from build123d import *

# Parameters (mm, degrees)
F1_R     = 4.7625
F2_DEPTH = 3.175
F3_R     = 12.7
F5_DEPTH = 336.55
F6_R     = 3.175


with BuildPart() as f2:
    # F1 (on Front) → F2 (new body)
    with BuildSketch(Plane.XZ):
        with BuildLine():
            Line((0, 438.028063), (0, 0))
            Line((0, 0), (336.55, 0))
            Line((336.55, 0), (336.55, 463.55))
            ThreePointArc((336.55, 463.55), (312.97337, 491.937548), (280.739907, 473.973298))
            Line((280.739907, 473.973298), (255.797312, 409.526661))
            Line((255.797312, 409.526661), (166.350515, 398.862006))
            Line((166.350515, 398.862006), (162.776801, 398.435916))
            Line((162.776801, 398.435916), (159.510839, 399.948027))
            Line((159.510839, 399.948027), (32.464507, 458.769359))
            ThreePointArc((32.464507, 458.769359), (10.552386, 457.288903), (0, 438.028063))
        make_face()
        with Locations((25.4, 419.1)):
            Circle(F1_R, mode=Mode.SUBTRACT)
        with Locations((309.557942, 388.978135)):
            Circle(F1_R, mode=Mode.SUBTRACT)
        with Locations((311.101928, 413.858754)):
            Circle(F1_R, mode=Mode.SUBTRACT)
        with Locations((310.471551, 438.779263)):
            Circle(F1_R, mode=Mode.SUBTRACT)
        with Locations((307.671607, 463.55)):
            Circle(F1_R, mode=Mode.SUBTRACT)
    extrude(amount=F2_DEPTH)

    # F3
    f3_edges = [f2.edges().sort_by_distance(p)[0] for p in [
        (162.776801, -1.5875, 398.435916),
        (255.797312, -1.5875, 409.526661),
    ]]
    fillet(f3_edges, radius=F3_R)

    # F4 (on Right) → F5 (join, through all)
    with BuildSketch(Plane.YZ):
        Polygon((0, 0), (-3.175, 0), (-3.175, -3.175), (50.8, -3.175), (50.8, 0), align=None)
    extrude(amount=F5_DEPTH)

    # F6
    f6_edges = [f2.edges().sort_by_distance(p)[0] for p in [
        (168.275, -3.175, -3.175),
    ]]
    fillet(f6_edges, radius=F6_R)


solid = f2.part
Can you work these out from the model? Positions are in its coordinate system, mm. A direction names the side the tool comes from. Coordinates: 2 decimals unless noted, no trailing zeros. Write each loop counter-clockwise with the first axis right and the second up, starting at its lowest first coordinate (ties: lowest second). Pieces come first, ordered by that corner, then holes. Notation, with made-up numbers: (-3.5, 87.5) -> (23.5, 87.5) arc R16 ccw to (23.5, 109.5) -> close; hole circle Ø7 at (-23.5, 0). An arc over 180 degrees is marked (long way). Write each question's results on one line, items separated by ' | '. Start each with the question number.
Q1. Imagine slicing it at D-D (x = 195). Write out the boundary of the cut face in (y, z) (3 decimals).
Q2. If I drill on probe 1 along Z at (x, y) = (201.5, 41) (3 decimals); probe 2 along X at (y, z) = (-1.7, 463.55), over which ranges is the centre line in solid material (lowest first)?
Q3. Imagine slicing it at B-B (z = 261). Write out the boundary of the cut face in (x, y) (3 decimals), then the cut area to 3 significant figures.
Q4. On a 3-axis mill with a long thin cutter (end or side, diameter ignored), from which of +Z, -Z, +X, -X, +Y, -Y can I reach the whole of each face in a straight line? I mean faces 1 (the face through (303.892, -1.565, 460.652)), 2 (the face through (166, 26, 0)). Say none if no direction works.
Q5. Imagine slicing it at A-A (x = 131.5). Write out the boundary of the cut face in (y, z) (3 decimals), then the cut area to 3 significant figures.
Q6. We'd pull the mould along Z, two halves only. Please class faces 3 (the face through (269.8, -1.57, 445.71)), 4 (the face through (24.37, -1.57, 414.45)), 5 (the face through (166, 0, 195)): +Z half, -Z half, draft (parallel to the pull), parting line (faces both ways), or undercut.
Q7. I'm going to push flat-ended pins straight in: pin 1 (8.5 mm diameter, centred on x = 309.56, z = 388.98, fed in from -Y); pin 2 (5 mm diameter, centred on x = 42.5, y = 33.5, fed in from +Z); pin 3 (3 mm diameter, centred on x = 180, z = 161.5, fed in from +Y). Where does each tip first touch, or does it pass through?
Taken from the geometry:
1) outline: (-3.175, 0) arc R3.175 ccw to (0, -3.175) -> (50.8, -3.175) -> (50.8, 0) -> (0, 0) -> (0, 402.278) -> (-3.175, 402.278) -> close
2) probe 1: z = -3.175 to 0 | probe 2: x = 276.71 to 302.91, 312.43 to 336.55
3) outline: (0, -3.175) -> (336.55, -3.175) -> (336.55, 0) -> (0, 0) -> close | area: 1,070 mm^2
4) face 1: +Y, -Y | face 2: +Z, +X, -X, +Y
5) outline: (-3.175, 0) arc R3.175 ccw to (0, -3.175) -> (50.8, -3.175) -> (50.8, 0) -> (0, 0) -> (0, 412.917) -> (-3.175, 412.917) -> close | area: 1,480 mm^2
6) face 3: +Z half | face 4: undercut | face 5: draft
7) pin 1: passes through | pin 2: stops at z = 0 | pin 3: stops at y = 0
